Read the model definition and answer for the solid it produces. Units are mm, in the model's axes. Face numbers are marked on the shaded views. A direction names the side the tool comes from. Round coordinates to 2 decimals unless told otherwise and drop trailing zeros. Write each loop counter-clockwise with the first axis right and the second up, starting at its lowest first coordinate (ties: lowest second). Pieces come first, ordered by that corner, then holes. Notation, with made-up numbers: (55, 63) -> (106, 63) arc R7 ccw to (106, 74) -> close; hole circle Ø6 at (62.25, 17.5). An arc over 180 degrees is marked (long way). Return JSON: item names as keys, results as strings. Group by question number.
(1) A cutting plane is placed at C-C on y = 11. Give the vertices of the cut face in (x, z), then the cut area to 3 significant figures.
(2) Given pin 1 (4 mm diameter, centred on x = -98, y = 42.5, fed in from +Z), flat-ended and moving along its own axis, determine where the tip first touches the part or whether it passes through.
(3) A cutting plane is placed at A-A on x = -12.5. Give the vertices of the cut face in (y, z), then the cut area to 3 significant figures.
(4) A cutting plane is placed at B-B on z = 8. Give the vertices of the cut face in (x, y), then the cut area to 3 significant figures.
(5) A cutting plane is placed at D-D on x = -91. Give the vertices of the cut face in (y, z).
(6) The mould has two halves that part along Y. Classify the marked faces 1, 2 and 3: released by +Y, released by -Y, zero draft, split by the parting line, or undercut.
(7) For the marked faces 4 and 5, determine the directions among +Z, -Z, +X, -X, +Y, -Y from which every point of the face is accessible in a straight line to the end or side of a thin tool.
(8) Straight lines are drawn through the part: line 1 (Y direction, x = -75.5, z = 11); line 2 (X direction, y = 53, z = 23); line 3 (Y direction, x = -17.5, z = 18.75). For each, find the intervals that lie inside material, in ascending order.
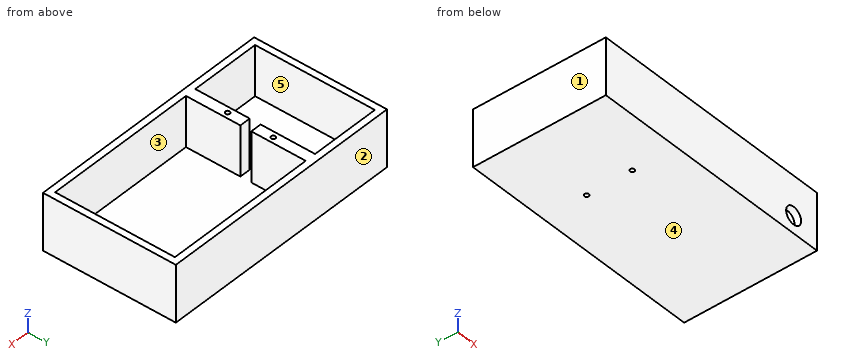
```python
from build123d import *

# Parameters (mm, degrees)
SKETCH1_W           = 113
SKETCH1_H           = 61
SKETCH1_W_2         = 70
SKETCH1_H_2         = 55
SKETCH1_W_3         = 32
BOSS_EXTRUDE1_DEPTH = 26
SKETCH2_W           = 70
SKETCH2_H           = 55
SKETCH2_W_2         = 32
BOSS_EXTRUDE2_DEPTH = 3
SKETCH3_W           = 23
SKETCH3_H           = 5
CUT_EXTRUDE1_DEPTH  = 5
SKETCH5_R           = 4
CUT_EXTRUDE3_DEPTH  = 10
SKETCH6_R           = 1
CUT_EXTRUDE4_DEPTH  = 30


with BuildPart() as part:
    # Sketch1 → Boss-Extrude1 (new body)
    with BuildSketch(Plane.XY):
        with Locations((-56.5, 30.5)):
            Rectangle(SKETCH1_W, SKETCH1_H)
        with Locations((-38, 30.5)):
            Rectangle(SKETCH1_W_2, SKETCH1_H_2, mode=Mode.SUBTRACT)
        with Locations((-94, 30.5)):
            Rectangle(SKETCH1_W_3, SKETCH1_H_2, mode=Mode.SUBTRACT)
    extrude(amount=BOSS_EXTRUDE1_DEPTH)

    # Sketch2 → Boss-Extrude2 (add)
    with BuildSketch(Plane(origin=(0, 0, 0), x_dir=(-1, 0, 0), z_dir=(0, 0, -1))):
        with Locations((38, 30.5)):
            Rectangle(SKETCH2_W, SKETCH2_H)
        with Locations((94, 30.5)):
            Rectangle(SKETCH2_W_2, SKETCH2_H)
    extrude(amount=-BOSS_EXTRUDE2_DEPTH)

    # Sketch3 → Cut-Extrude1 (cut)
    with BuildSketch(Plane(origin=(-73, 0, 0), x_dir=(0, 0, -1), z_dir=(1, 0, 0))):
        with Locations((-14.5, 30.5)):
            Rectangle(SKETCH3_W, SKETCH3_H)
    extrude(amount=-CUT_EXTRUDE1_DEPTH, mode=Mode.SUBTRACT)

    # Sketch5 → Cut-Extrude3 (cut)
    with BuildSketch(Plane(origin=(0, 0, 0), x_dir=(-1, 0, 0), z_dir=(0, -1, 0))):
        with Locations(Location((12.5, -8, 0), (0, 0, 90))):
            Circle(SKETCH5_R)
    extrude(amount=-CUT_EXTRUDE3_DEPTH, mode=Mode.SUBTRACT)

    # Sketch6 → Cut-Extrude4 (cut)
    with BuildSketch(Plane.XY.offset(26)):
        with Locations((-75.5, 41)):
            Circle(SKETCH6_R)
        with Locations((-75.5, 20)):
            Circle(SKETCH6_R)
    extrude(amount=-CUT_EXTRUDE4_DEPTH, mode=Mode.SUBTRACT)


solid = part.part
```
Checks:
{
 "1": {"outline": "(-113, 0) -> (0, 0) -> (0, 26) -> (-3, 26) -> (-3, 3) -> (-73, 3) -> (-73, 26) -> (-78, 26) -> (-78, 3) -> (-110, 3) -> (-110, 26) -> (-113, 26) -> close", "area": "592 mm^2"},
 "2": {"pin 1": "stops at z = 3"},
 "3": {"outline": "(0, 0) -> (61, 0) -> (61, 26) -> (58, 26) -> (58, 3) -> (3, 3) -> (3, 4) -> (0, 4) -> close; (0, 12) -> (3, 12) -> (3, 26) -> (0, 26) -> close", "area": "297 mm^2"},
 "4": {"outline": "(-113, 0) -> (-16.5, 0) -> (-16.5, 3) -> (-73, 3) -> (-73, 28) -> (-78, 28) -> (-78, 3) -> (-110, 3) -> (-110, 58) -> (-78, 58) -> (-78, 33) -> (-73, 33) -> (-73, 58) -> (-3, 58) -> (-3, 3) -> (-8.5, 3) -> (-8.5, 0) -> (0, 0) -> (0, 61) -> (-113, 61) -> close; hole circle Ø2 at (-75.5, 20); hole circle Ø2 at (-75.5, 41)", "area": "1,230 mm^2"},
 "5": {"outline": "(0, 0) -> (61, 0) -> (61, 26) -> (58, 26) -> (58, 3) -> (3, 3) -> (3, 26) -> (0, 26) -> close"},
 "6": {"face 1": "zero draft", "face 2": "released by +Y", "face 3": "undercut"},
 "7": {"face 4": "-Z, +X, -X, +Y, -Y", "face 5": "+Z"},
 "8": {"line 1": "y = 0 to 19, 21 to 28, 33 to 40, 42 to 61", "line 2": "x = -113 to -110, -78 to -73, -3 to 0", "line 3": "y = 0 to 3, 58 to 61"}
}
